```python
from build123d import *

# Parameters (mm, degrees)
F0_R     = 35
F0_R_2   = 18.75
F1_DEPTH = 30
F0_R_3   = 6.75
F0_R_4   = 7.5
F2_DEPTH = 85
F3_R     = 5


with BuildPart() as f1:
    # F0 (on Top) → F1 (new body)
    with BuildSketch(Plane.XY):
        Circle(F0_R)
        Circle(F0_R_2, mode=Mode.SUBTRACT)
    extrude(amount=F1_DEPTH)

    # F0 (on Top) → F2 (join)
    with BuildSketch(Plane.XY):
        Circle(F0_R_2)
        with Locations((-9.115429, 0)):
            Circle(F0_R_3, mode=Mode.SUBTRACT)
        with Locations((9.25153, 0)):
            Circle(F0_R_4, mode=Mode.SUBTRACT)
    extrude(amount=F2_DEPTH)

    # F3
    f3_edges = [f1.edges().sort_by_distance(p)[0] for p in [
        (-35, 0, 0),
    ]]
    fillet(f3_edges, radius=F3_R)


solid = f1.part
```
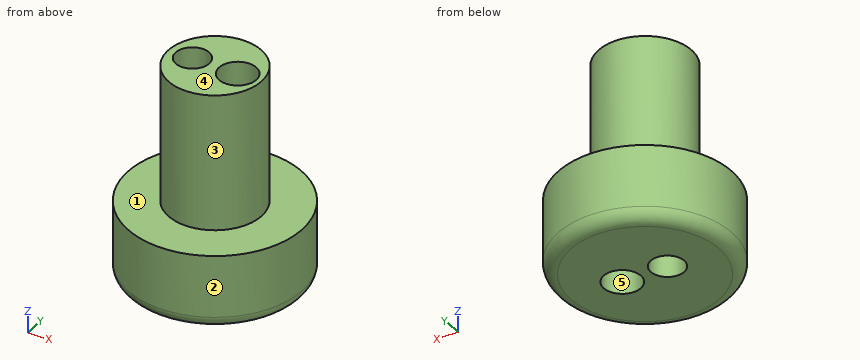
The listing builds one solid part. Answer for the finished solid, in the listing's coordinates (mm). Face numbers are marked on the shaded views. A direction names the side the tool comes from. Give positions to 0.01 mm unless a question says otherwise; leave off trailing zeros. Write each loop counter-clockwise with the first axis right and the second up, starting at its lowest first coordinate (ties: lowest second). Pieces come first, ordered by that corner, then holes. Notation, with made-up numbers: M 6.5,3 L 58.5,3 A30 cw 58.5,27 Z; hole C 79,36.5 d7. An arc over 180 degrees is marked long. Write each question's results on one line, items separated by ' | '.
Q1. Section A-A, the plane y = 0 is taken. Write down the section's boundary in (x, z), then the cut area to 3 significant figures.
Output values:
outline: M -35,5 A5 ccw -30,0 L -15.87,0 L -15.87,85 L -18.75,85 L -18.75,30 L -35,30 Z; M -2.37,0 L 1.75,0 L 1.75,85 L -2.37,85 Z; M 16.75,0 L 30,0 A5 ccw 35,5 L 35,30 L 18.75,30 L 18.75,85 L 16.75,85 Z | area: 1,730 mm2
Q2. Flat-ended cylindrical pins translate along their axes: P1, Ø5, axis at y = 12.5, z = 26, coming from the -X side; P2, Ø2, axis at y = -21, z = 56.5, coming from the +X side; P3, Ø8, axis at y = 16.5, z = 20, coming from the +X side; P4, Ø1.5, axis at x = 20, z = 18, coming from the +Y side. Find the tip coordinate at first contact, or state that the pin passes through.
Output values:
P1: x = -33.54 | P2: through | P3: x = 32.69 | P4: y = 29.23
Q3. A tool of negligible diameter and unlimited length cuts with its end or side. For the marked faces 1 and 2, from which of +Z, -Z, +X, -X, +Y, -Y can it reach the whole face along a straight path? Write none if from no direction.
Output values:
face 1: +Z | face 2: +Z, -Z
Q4. Section C-C, the plane z = 37 is taken. Write down the section's boundary in (x, y).
Output values:
outline: C 0,0 d37.5; hole C -9.12,0 d13.5; hole C 9.25,0 d15
Q5. For a pull along X with two mould halves and no side action, classify the marked faces 3, 4 and 5 as released by +X, released by -X, zero draft, split by the parting line, or undercut.
Output values:
face 3: split by the parting line | face 4: zero draft | face 5: undercut
Q6. Section B-B, the plane x = 0 is taken. Write down the section's boundary in (y, z), then the cut area to 3 significant figures.
Output values:
outline: M -35,5 A5 ccw -30,0 L 30,0 A5 ccw 35,5 L 35,30 L 18.75,30 L 18.75,85 L -18.75,85 L -18.75,30 L -35,30 Z | area: 4,150 mm2
Q7. Consider L1, parallel to X at y = 3, z = 47; L2, parallel to Z at x = 15, y = 20; L3, parallel to Y at x = 6, z = 72. Determine where each line is inside the solid, lowest interval first. Write a range as from..to.
Output values:
L1: -18.51..-15.16, -3.07..2.38, 16.13..18.51 | L2: 0..30 | L3: -17.76..-6.76, 6.76..17.76
